Could you check a few things on this model? Use its own coordinates, in mm. Round coordinates to 2 decimals unless told otherwise and drop trailing zeros. Write each loop counter-clockwise with the first axis right and the second up, starting at its lowest first coordinate (ties: lowest second). Pieces come first, ordered by that corner, then holes. Notation, with made-up numbers: (8, 60) - (33, 60) arc R20 cw to (33, 98) - close; hole circle Ø9 at (10.25, 4.25). An arc over 180 degrees is marked (long way). Put each result on its own line as item: value.
from build123d import *

# Parameters (mm, degrees)
OUTER_CUT_DEPTH    = 1.5875
SLOTS_DEPTH        = 195.298586266
SKETCH3_R          = 1.5875
MOUNT_HOLES_DEPTH  = 195.298586266
SKETCH4_R          = 1.5875
CUT_EXTRUDE1_DEPTH = 195.298586266


with BuildPart() as part:
    # Sketch1 → Outer Cut (new, symmetric)
    with BuildSketch(Plane(origin=(0, 0, 0), x_dir=(0, 0, -1), z_dir=(1, 0, 0))):
        with BuildLine():
            Line((-184.15, -38.1), (184.15, -38.1))
            ThreePointArc((184.15, -38.1), (188.640128061, -36.240128061), (190.5, -31.75))
            Line((190.5, -31.75), (190.5, 31.75))
            ThreePointArc((190.5, 31.75), (188.640128061, 36.240128061), (184.15, 38.1))
            Line((184.15, 38.1), (-184.15, 38.1))
            ThreePointArc((-184.15, 38.1), (-188.640128061, 36.240128061), (-190.5, 31.75))
            Line((-190.5, 31.75), (-190.5, -31.75))
            ThreePointArc((-190.5, -31.75), (-188.640128061, -36.240128061), (-184.15, -38.1))
        make_face()
    extrude(amount=OUTER_CUT_DEPTH, both=True)

    # Sketch2 → Slots (cut, through all)
    with BuildSketch(Plane(origin=(1.5875, 0, 0), x_dir=(0, 0, -1), z_dir=(1, 0, 0))):
        with BuildLine():
            Line((-177.8, 22.225), (177.8, 22.225))
            ThreePointArc((177.8, 22.225), (180.975, 19.05), (177.8, 15.875))
            Line((177.8, 15.875), (-177.8, 15.875))
            ThreePointArc((-177.8, 15.875), (-180.975, 19.05), (-177.8, 22.225))
        make_face()
        with BuildLine():
            Line((-177.8, -22.225), (177.8, -22.225))
            ThreePointArc((177.8, -22.225), (180.975, -19.05), (177.8, -15.875))
            Line((177.8, -15.875), (-177.8, -15.875))
            ThreePointArc((-177.8, -15.875), (-180.975, -19.05), (-177.8, -22.225))
        make_face()
    extrude(amount=-SLOTS_DEPTH, mode=Mode.SUBTRACT)

    # Sketch3 → Mount Holes (cut, through all)
    with BuildSketch(Plane(origin=(1.5875, 0, 0), x_dir=(0, 0, -1), z_dir=(1, 0, 0))):
        with Locations((-184.15, 31.75)):
            Circle(SKETCH3_R)
        with Locations((-120.65, 31.75)):
            Circle(SKETCH3_R)
        with Locations(Location((-120.65, -31.75, 0), (0, 0, 180))):
            Circle(SKETCH3_R)
        with Locations(Location((-184.15, -31.75, 0), (0, 0, 180))):
            Circle(SKETCH3_R)
        with Locations((-184.15, 0)):
            Circle(SKETCH3_R)
        with Locations((-120.65, 0)):
            Circle(SKETCH3_R)
    extrude(amount=-MOUNT_HOLES_DEPTH, mode=Mode.SUBTRACT)

    # Sketch4 → Cut-Extrude1 (cut, through all)
    with BuildSketch(Plane(origin=(1.5875, 0, 0), x_dir=(0, 0, -1), z_dir=(1, 0, 0))):
        with Locations((184.15, 31.75)):
            Circle(SKETCH4_R)
        with Locations((174.625, 31.75)):
            Circle(SKETCH4_R)
        with Locations(Location((174.625, -31.75, 0), (0, 0, 180))):
            Circle(SKETCH4_R)
        with Locations(Location((184.15, -31.75, 0), (0, 0, 180))):
            Circle(SKETCH4_R)
    extrude(amount=-CUT_EXTRUDE1_DEPTH, mode=Mode.SUBTRACT)


solid = part.part
(1) Imagine slicing it at B-B, the plane x = 1. Give the number of separate pieces and of enclosed holes in the cut face, then the cut area to 3 significant figures.
Values found:
separate pieces: 1
enclosed holes: 12
area: 24,300 mm^2
(2) Imagine slicing it at A-A, the plane z = 141.5. List the corners of the cut face in (x, y) for me (1 decimal), then the cut area to 3 significant figures.
Values found:
outline: (-1.6, -38.1) - (1.6, -38.1) - (1.6, -22.2) - (-1.6, -22.2) - close; (-1.6, -15.9) - (1.6, -15.9) - (1.6, 15.9) - (-1.6, 15.9) - close; (-1.6, 22.2) - (1.6, 22.2) - (1.6, 38.1) - (-1.6, 38.1) - close
area: 202 mm^2
(3) Imagine slicing it at C-C, the plane y = -19.05. List the corners of the cut face in (x, z) for me (1 decimal), then the cut area to 3 significant figures.
Values found:
outline: (-1.6, -190.5) - (1.6, -190.5) - (1.6, -181) - (-1.6, -181) - close; (-1.6, 181) - (1.6, 181) - (1.6, 190.5) - (-1.6, 190.5) - close
area: 60.5 mm^2
(4) Please list where these lines run through material, in increasing order: probe 1 along Z at (x, y) = (0.3, -31.75); probe 2 along Y at (x, z) = (0.9, 104) (3 decimals); probe 3 along Z at (x, y) = (-0.05, 32.5). Write a range as from..to.
Values found:
probe 1: z = -190.5..-185.74, -182.56..-176.21, -173.04..119.06, 122.24..182.56, 185.74..190.5
probe 2: y = -38.1..-22.225, -15.875..15.875, 22.225..38.1
probe 3: z = -190.46..-185.55, -182.75..-176.02, -173.23..119.25, 122.05..182.75, 185.55..190.46
(5) I'm going to push flat-ended pins straight in: pin 1 (2.5 mm diameter, centred on y = -31.75, z = -174.625, fed in from -X); pin 2 (2 mm diameter, centred on y = 0, z = 122, fed in from +X). Where does each tip first touch, or does it pass through?
Values found:
pin 1: passes through
pin 2: stops at x = 1.59
